Autodesk Inventor part; units mm, degrees
ref_plane "YZ Plane" through (0, 0, 0) normal (1, 0, 0) x (0, 1, 0)
ref_plane "XZ Plane" through (0, 0, 0) normal (0, 1, 0) x (-1, 0, 0)
ref_plane "XY Plane" through (0, 0, 0) normal (0, 0, 1) x (1, 0, 0)
sketch "Sketch1" plane through (0, 0, 0) normal (0, 0, 1) x (1, 0, 0)
  line L0 (0, 0) -> (-35.2056, 0)
  line L1 (-35.2056, 0) -> (-65.5234, -36.1314)
  line L2 (-65.5234, -36.1314) -> (-73.1839, -29.7035)
  line L3 (-73.1839, -29.7035) -> (-39.8687, 10)
  line L4 (-39.8687, 10) -> (0, 10)
  line L5 (0, 10) -> (0, 0)
  circle A0 centre (-66.1397, -29.0872) radius 3
  circle A1 centre (-5, 5) radius 3.25
  line L6 (0, 5) -> (-37.5371, 5) construction
  line L7 (-37.5371, 5) -> (-69.3536, -32.9174) construction
  line L8 (0, 0) -> (-65.5234, -36.1314) construction
  line L9 (0, 10) -> (5, 10)
  line L10 (5, 10) -> (5, 0)
  line L11 (5, 0) -> (0, 0)
  line L12 (0, 0) -> (0, 10)
  dimension "d0" = 10
  dimension "d1" = 6
  dimension "d2" = 6.5
  dimension "d3" = 5
  dimension "d4" = 5
  dimension "d5" = 70
  dimension "d26" = 50
  dimension "d28" = 17
  dimension "d37" = 5
extrude "Extrusion1" add sketch "Sketch1" along normal blind 9.3
fillet "Fillet1" radius 5 3 edges at (-73.1839, -29.7035, 4.65) (-65.5234, -36.1314, 4.65) (-35.2056, 0, 4.65)
sketch "Sketch5" plane through (0, 0, 0) normal (0, 0, -1) x (-1, 0, 0)
  circle A0 centre (5, 5) radius 3.25
  point P0 (0, 0)
  point P1 (12, 5)
  point P2 (-2, 5)
  dimension "d29" = 7
  dimension "d38" = 7
hole "Hole1" at (-12, 5, 0) at (2, 5, 0) direction (0, 0, 1) diameter 2.459 end through all
sketch "Sketch4" plane through (0, 0, 9.3) normal (0, 0, 1) x (1, 0, 0)
  line L0 (0, 0) -> (-30, 0)
  line L1 (-30, 0) -> (-30, 10)
  line L2 (-30, 10) -> (0, 10)
  line L3 (0, 10) -> (0, 0)
  line L4 (0, 10) -> (5, 10)
  line L5 (5, 10) -> (5, 0)
  line L6 (5, 0) -> (0, 0)
  line L7 (0, 0) -> (0, 10)
  dimension "d20" = 30
extrude "Extrusion4" cut sketch "Sketch4" against normal blind 4
sketch "Sketch6" plane through (0, 0, 9.3) normal (0, 0, 1) x (1, 0, 0)
  line L0 (-3.6029, 27.6633) -> (-80.9851, -10.0258)
  line L1 (-80.9851, -10.0258) -> (-68.4455, -35.7718)
  line L2 (-68.4455, -35.7718) -> (8.9367, 1.9174)
  line L3 (8.9367, 1.9174) -> (-3.6029, 27.6633)
  arc A0 (-69.9699, -25.8733) -> (-62.3095, -32.3011) centre (-66.1397, -29.0872) ccw
  line L4 (-83.6105, -9.1202) -> (-2.6973, 30.2887)
  line L5 (-2.6973, 30.2887) -> (11.5621, 1.0117)
  line L6 (11.5621, 1.0117) -> (-69.3511, -38.3971)
  line L7 (-69.3511, -38.3971) -> (-83.6105, -9.1202)
  point P0 (0, 0)
  point P1 (5, 10)
  point P2 (-39.8687, 10)
  point P3 (5, 0)
  dimension "d39" = 90
  dimension "d40" = 32.5648
  dimension "d41" = 1.9638
equation "\"d3\" = 0.5 * d0"
equation "\"d4\" = 0.5 * d0"
properties part number "Servo_Strut_v2" material "Steel, Carbon"
Verification items for the finished model (mm, model axes). A direction names the side the tool comes from. Give positions to 0.01 mm unless a question says otherwise; leave off trailing zeros. Write each loop counter-clockwise with the first axis right and the second up, starting at its lowest first coordinate (ties: lowest second). Pieces come first, ordered by that corner, then holes. Notation, with made-up numbers: M 41.25,-26.75 L 92.25,-26.75 A8 ccw 92.25,-14.75 Z; hole C 8,72.5 d6. An arc over 180 degrees is marked long. Use CSV: the item, a comma, the result in double quotes.
1) Material ranges on line 1 along X through (y, z) = (5, 4.1); line 2 along Y through (x, z) = (-12, 1.45); line 3 along Y through (x, z) = (-31.5, 4.75), recorded low to high.
Final values:
line 1,"-44.06 to -13.23, -10.77 to -8.25, -1.75 to 0.77, 3.23 to 5"
line 2,"0 to 3.77, 6.23 to 10"
line 3,"0 to 10"
2) Cross-section at A-A (x = -12). Enter the section's corners in (y, z), plus the area to 3 significant figures.
Final values:
outline,"M 0,0 L 3.77,0 L 3.77,5.3 L 0,5.3 Z; M 6.23,0 L 10,0 L 10,5.3 L 6.23,5.3 Z"
area,"40.0 mm²"
3) Go/stop test with flat-tipped pins: pin 1 Ø2 at (x, z) = (-34, 6.5) entering from -Y; pin 2 Ø5 at (x, y) = (-5.5, 3.5) entering from +Z; pin 3 Ø1 at (y, z) = (-10, 7) entering from -X. Record where each tip stops, or that it passes through.
Final values:
pin 1,"y = -0.47"
pin 2,"z = 5.3"
pin 3,"x = -57.07"
4) Cross-section at D-D (x = -25.5). Enter the section's corners in (y, z).
Final values:
outline,"M 0,0 L 10,0 L 10,5.3 L 0,5.3 Z"
5) Cross-section at B-B (y = 5). Enter the section's corners in (x, z), plus the area to 3 significant figures.
Final values:
outline,"M -44.06,0 L -13.23,0 L -13.23,5.3 L -30,5.3 L -30,9.3 L -44.06,9.3 Z; M -10.77,0 L -8.25,0 L -8.25,5.3 L -10.77,5.3 Z; M -1.75,0 L 0.77,0 L 0.77,5.3 L -1.75,5.3 Z; M 3.23,0 L 5,0 L 5,5.3 L 3.23,5.3 Z"
area,"256 mm²"
6) Access from +Z, -Z, +X, -X, +Y, -Y to the whole of each face (thin tool, end or side, straight path). Record for faces 4 (the face through (-3.5, 7.883, 2.613)), 5 (the face through (-13, 4, 5.3)), 6 (the face through (-14, 0, 3)).
Final values:
face 4,"+Z, -Z"
face 5,"+Z, +X, +Y, -Y"
face 6,"+Z, -Z, +X, -Y"
7) Release check for a two-part mould opening along X. For faces 1 (the face through (1.95, 3.77, 2.69)), 2 (the face through (-71.125, -29.468, 4.715)), 3 (the face through (-34.959, -0.456, 4.715)) record: released by +X, released by -X, zero draft, split by the parting line, or undercut.
Final values:
face 1,"undercut"
face 2,"released by -X"
face 3,"released by +X"
